Geometry: final body of the model. Coordinates: model frame, mm. A direction names the side the tool comes from. Give positions to 0.01 mm unless a question says otherwise; leave off trailing zeros. Write each loop counter-clockwise with the first axis right and the second up, starting at its lowest first coordinate (ties: lowest second). Pieces come first, ordered by that corner, then holes. Notation, with made-up numbers: (-19, 17) - (14, 17) arc R17 cw to (14, 45) - close; hole circle Ø10 at (58.25, 65.25). An arc over 180 degrees is marked (long way). Return JSON: item names as keys, results as strings.
from build123d import *

# Parameters (mm, degrees)
ESQUISSE1_W             = 40.9
ESQUISSE1_H             = 5
ESQUISSE1_W_2           = 8
ESQUISSE1_H_2           = 30
ESQUISSE1_R             = 2
BOSS_EXTRU_1_DEPTH      = 9
ESQUISSE2_R             = 1.8
ENL_V_MAT_EXTRU_1_DEPTH = 9


with BuildPart() as part:
    # Esquisse1 → Boss.-Extru.1 (new body)
    # profile 1 of 3: a face of its own
    with BuildSketch(Plane.XY):
        with Locations((28.45, 2.5)):
            Rectangle(ESQUISSE1_W, ESQUISSE1_H)
    # profile 2 of 3: a face of its own
    with BuildSketch(Plane.XY):
        with Locations((4, 15)):
            Rectangle(ESQUISSE1_W_2, ESQUISSE1_H_2)
        with Locations((4.15, 15)):
            Circle(ESQUISSE1_R, mode=Mode.SUBTRACT)
        with Locations((4.15, 25)):
            Circle(ESQUISSE1_R, mode=Mode.SUBTRACT)
    # profile 3 of 3: a face of its own
    with BuildSketch(Plane.XY):
        Polygon((48.9, 5), (48.9, 0), (56.9, 0), (56.9, 30), (48.9, 30), align=None)
        with Locations((52.75, 15)):
            Circle(ESQUISSE1_R, mode=Mode.SUBTRACT)
        with Locations((52.75, 25)):
            Circle(ESQUISSE1_R, mode=Mode.SUBTRACT)
    extrude(amount=BOSS_EXTRU_1_DEPTH)

    # Esquisse2 → Enlèv. mat.-Extru.1 (cut)
    with BuildSketch(Plane.XZ):
        with Locations((18.45, 4.5)):
            Circle(ESQUISSE2_R)
        with Locations((38.45, 4.5)):
            Circle(ESQUISSE2_R)
    extrude(amount=-ENL_V_MAT_EXTRU_1_DEPTH, mode=Mode.SUBTRACT)


solid = part.part
Q1. Mould query, pull axis Z, two halves, no side actions, for faces 3 (the flat face through (28, 4, 0)), 4 (the flat face through (4, 30, 4)), 5 (the cylindrical face through (16.65, 2.46, 4.58)). Classes: pulls with the +Z half, pulls with the -Z half, needs draft (parallel to the pull), parting line crosses it, or undercut.
Answer key:
{"face 3": "pulls with the -Z half", "face 4": "needs draft", "face 5": "undercut"}
Q2. Set-up query: faces 1 (the flat face through (0, 15, 4)), 2 (the flat face through (48.9, 18, 4)). Return all of +Z, -Z, +X, -X, +Y, -Y with unobstructed straight access to the full face (end or side cutting, diameter ignored); none if empty.
Answer key:
{"face 1": "+Z, -Z, -X, +Y, -Y", "face 2": "+Z, -Z, +Y"}
Q3. Pin query (flat end, axial travel): P1, Ø4, axis at x = 18.45, z = 4.5, coming from the +Y side. Return the tip coordinate at first contact, or that it passes through.
Answer key:
{"P1": "stops at y = 5"}
Q4. Section query C-C, the plane x = 4.15. Return the cut outline in (y, z).
Answer key:
{"outline": "(0, 0) - (13, 0) - (13, 9) - (0, 9) - close; (17, 0) - (23, 0) - (23, 9) - (17, 9) - close; (27, 0) - (30, 0) - (30, 9) - (27, 9) - close"}
Q5. Section query A-A, the plane z = 4.5. Return the cut outline in (x, y), plus the area to 3 significant figures.
Answer key:
{"outline": "(0, 0) - (16.65, 0) - (16.65, 5) - (8, 5) - (8, 30) - (0, 30) - close; (20.25, 0) - (36.65, 0) - (36.65, 5) - (20.25, 5) - close; (40.25, 0) - (56.9, 0) - (56.9, 30) - (48.9, 30) - (48.9, 5) - (40.25, 5) - close; hole circle Ø4 at (4.15, 15); hole circle Ø4 at (4.15, 25); hole circle Ø4 at (52.75, 15); hole circle Ø4 at (52.75, 25)", "area": "598 mm^2"}
Q6. Section query B-B, the plane y = 21.25. Return the cut outline in (x, z), plus the area to 3 significant figures.
Answer key:
{"outline": "(0, 0) - (8, 0) - (8, 9) - (0, 9) - close; (48.9, 0) - (56.9, 0) - (56.9, 9) - (48.9, 9) - close", "area": "144 mm^2"}
Q7. Section query D-D, the plane y = 15. Return the cut outline in (x, z).
Answer key:
{"outline": "(0, 0) - (2.15, 0) - (2.15, 9) - (0, 9) - close; (6.15, 0) - (8, 0) - (8, 9) - (6.15, 9) - close; (48.9, 0) - (50.75, 0) - (50.75, 9) - (48.9, 9) - close; (54.75, 0) - (56.9, 0) - (56.9, 9) - (54.75, 9) - close"}
Q8. Material intervals for probe 1 along Y at (x, z) = (52.75, 5); probe 2 along X at (y, z) = (13.25, 3.75); probe 3 along X at (y, z) = (18.75, 5), sorted ascending. Write a range as [from, to].
Answer key:
{"probe 1": "y = [0, 13], [17, 23], [27, 30]", "probe 2": "x = [0, 3.18], [5.12, 8], [48.9, 51.78], [53.72, 56.9]", "probe 3": "x = [0, 8], [48.9, 56.9]"}
